from build123d import *

# Parameters (mm, degrees)
F0_W        = 7
F0_H        = 7
F0_W_2      = 1.15
F0_H_2      = 1.15
F1_DEPTH    = 6
F2_SIZE     = 0.1
F3_T1_DEPTH = 14.6069618105
F3_T3_DEPTH = 14.6069618105
F3_T5_DEPTH = 14.6069618105
F3_T7_DEPTH = 14.6069618105
F6_D        = 3
F6_DEPTH    = 6
F6_TIP      = 0.9012909285
F8_DEPTH    = 3.5
F9_SIZE     = 0.3


# Not quite as in the source:
# - a fillet or chamfer that OpenCascade refuses, or shapes differently, is made with other operations: its cross-section is extruded or revolved along the edge and cut away or added


with BuildPart() as f1:
    # F0 (on Front) → F1 (new body)
    with BuildSketch(Plane.XZ):
        Rectangle(F0_W, F0_H)
        with Locations((-2.54, -2.54)):
            Rectangle(F0_W_2, F0_H_2, mode=Mode.SUBTRACT)
        with Locations((0, -2.54)):
            Rectangle(F0_W_2, F0_H_2, mode=Mode.SUBTRACT)
        with Locations((2.54, -2.54)):
            Rectangle(F0_W_2, F0_H_2, mode=Mode.SUBTRACT)
        with Locations((-2.54, 2.54)):
            Rectangle(F0_W_2, F0_H_2, mode=Mode.SUBTRACT)
        with Locations((0, 2.54)):
            Rectangle(F0_W_2, F0_H_2, mode=Mode.SUBTRACT)
        with Locations((2.54, 2.54)):
            Rectangle(F0_W_2, F0_H_2, mode=Mode.SUBTRACT)
        with Locations((-2.54, -2.54)):
            Rectangle(F0_W_2, F0_H_2)
        with Locations((0, -2.54)):
            Rectangle(F0_W_2, F0_H_2)
        with Locations((0, 2.54)):
            Rectangle(F0_W_2, F0_H_2)
        with Locations((-2.54, 2.54)):
            Rectangle(F0_W_2, F0_H_2)
        with Locations((2.54, 2.54)):
            Rectangle(F0_W_2, F0_H_2)
        with Locations((2.54, -2.54)):
            Rectangle(F0_W_2, F0_H_2)
    extrude(amount=F1_DEPTH)

    # F2
    f2_edges = [f1.edges().sort_by_distance(p)[0] for p in [
        (3.5, -6, 0),
        (0, -6, 3.5),
        (-3.5, -6, 0),
        (0, -6, -3.5),
    ]]
    chamfer(f2_edges, length=F2_SIZE)

    # F3: fillet of radius 5 on 4 edges, made by hand

    # F3_s2 → F3_t1 (cut)
    with BuildSketch(Plane(origin=(4.5333333333, 4.5333333333, 4.5333333333), x_dir=(0.7071067812, -0.7071067812, 0), z_dir=(-0.5773502692, -0.5773502692, -0.5773502692))):
        with BuildLine():
            ThreePointArc((4.1468037432, 5.2809096033), (5.9769307621, 3.4507825844), (6.6468037432, 0.9507825844))
            Line((6.6468037432, 0.9507825844), (6.6468037432, 3.8375339304))
            Line((6.6468037432, 3.8375339304), (4.1468037432, 5.2809096033))
        make_face()
    extrude(amount=F3_T1_DEPTH, mode=Mode.SUBTRACT)

    # F3_s4 → F3_t3 (cut)
    with BuildSketch(Plane(origin=(-4.5333333333, 4.5333333333, 4.5333333333), x_dir=(0.7071067812, 0.7071067812, 0), z_dir=(0.5773502692, -0.5773502692, -0.5773502692))):
        with BuildLine():
            ThreePointArc((-4.1468037432, 5.2809096033), (-5.9769307621, 3.4507825844), (-6.6468037432, 0.9507825844))
            Line((-6.6468037432, 0.9507825844), (-6.6468037432, 3.8375339304))
            Line((-6.6468037432, 3.8375339304), (-4.1468037432, 5.2809096033))
        make_face()
    extrude(amount=F3_T3_DEPTH, mode=Mode.SUBTRACT)

    # F3_s6 → F3_t5 (cut)
    with BuildSketch(Plane(origin=(4.5333333333, 4.5333333333, -4.5333333333), x_dir=(0.7071067812, -0.7071067812, 0), z_dir=(-0.5773502692, -0.5773502692, 0.5773502692))):
        with BuildLine():
            ThreePointArc((6.6468037432, -0.9507825844), (5.9769307621, -3.4507825844), (4.1468037432, -5.2809096033))
            Line((4.1468037432, -5.2809096033), (6.6468037432, -3.8375339304))
            Line((6.6468037432, -3.8375339304), (6.6468037432, -0.9507825844))
        make_face()
    extrude(amount=F3_T5_DEPTH, mode=Mode.SUBTRACT)

    # F3_s8 → F3_t7 (cut)
    with BuildSketch(Plane(origin=(-4.5333333333, 4.5333333333, -4.5333333333), x_dir=(0.7071067812, 0.7071067812, 0), z_dir=(0.5773502692, -0.5773502692, 0.5773502692))):
        with BuildLine():
            ThreePointArc((-6.6468037432, -0.9507825844), (-5.9769307621, -3.4507825844), (-4.1468037432, -5.2809096033))
            Line((-4.1468037432, -5.2809096033), (-6.6468037432, -3.8375339304))
            Line((-6.6468037432, -3.8375339304), (-6.6468037432, -0.9507825844))
        make_face()
    extrude(amount=F3_T7_DEPTH, mode=Mode.SUBTRACT)

    # F6
    with Locations(Plane.XZ.offset(6)):
        with Locations((0, 0)):
            Hole(F6_D / 2, depth=F6_DEPTH)
            with Locations((0, 0, -(F6_DEPTH + F6_TIP / 2))):  # 118° drill point
                Cone(0, F6_D / 2, F6_TIP, mode=Mode.SUBTRACT)

    # F0 (on Front) → F8 (join)
    with BuildSketch(Plane.XZ):
        with Locations((2.54, 2.54)):
            Rectangle(F0_W_2, F0_H_2)
        with Locations((0, 2.54)):
            Rectangle(F0_W_2, F0_H_2)
        with Locations((-2.54, 2.54)):
            Rectangle(F0_W_2, F0_H_2)
        with Locations((-2.54, -2.54)):
            Rectangle(F0_W_2, F0_H_2)
        with Locations((0, -2.54)):
            Rectangle(F0_W_2, F0_H_2)
        with Locations((2.54, -2.54)):
            Rectangle(F0_W_2, F0_H_2)
    extrude(amount=-F8_DEPTH)

    # F9
    f9_edges = [f1.edges().sort_by_distance(p)[0] for p in [
        (2.54, 3.5, -3.115),
        (1.965, 3.5, -2.54),
        (3.115, 3.5, -2.54),
        (2.54, 3.5, -1.965),
        (0.575, 3.5, -2.54),
        (0, 3.5, -3.115),
        (-0.575, 3.5, -2.54),
        (0, 3.5, -1.965),
        (-1.965, 3.5, -2.54),
        (-2.54, 3.5, -1.965),
        (-3.115, 3.5, -2.54),
        (-2.54, 3.5, -3.115),
        (3.115, 3.5, 2.54),
        (2.54, 3.5, 1.965),
        (1.965, 3.5, 2.54),
        (2.54, 3.5, 3.115),
        (0.575, 3.5, 2.54),
        (0, 3.5, 3.115),
        (-0.575, 3.5, 2.54),
        (0, 3.5, 1.965),
        (-1.965, 3.5, 2.54),
        (-2.54, 3.5, 1.965),
        (-3.115, 3.5, 2.54),
        (-2.54, 3.5, 3.115),
    ]]
    chamfer(f9_edges, length=F9_SIZE)


solid = f1.part
Input: part model. Units: mm. Frame: model coordinates. A direction names the side the tool comes from. Coordinates: 2 decimals unless noted, no trailing zeros. Loops run counter-clockwise (first coordinate to the right, second up) from the corner with the lowest first, then second, coordinate; pieces in that order, holes last.
(1) Set-up query: faces 5 (the face through (3.115, 1.6, 2.5)), 6 (the face through (1.965, 1.6, -2.5)), 7 (the face through (-3.115, 1.6, 2.5)), 8 (the face through (2.5, 1.6, 1.965)). Return all of +Z, -Z, +X, -X, +Y, -Y with unobstructed straight access to the full face (end or side cutting, diameter ignored); none if empty.
(2) Pull-direction query (X, two-part tool) for faces 1 (the face through (0.575, 1.6, -2.5)), 2 (the face through (3.115, 1.6, -2.5)), 3 (the face through (-2.72, -5.724, 2.737)), 4 (the face through (-2.5, 1.6, -1.965)); classes: released by +X, released by -X, zero draft, split by the parting line, or undercut.
(3) First-contact query: pin 1 Ø0.6 at (y, z) = (1, 2.5) entering from +X (3 decimals); pin 2 Ø0.9 at (x, y) = (0, 1.5) entering from +Z (3 decimals); pin 3 Ø0.6 at (y, z) = (2, 2.5) entering from -X (3 decimals). Flat tips, straight axial feed; report the tip coordinate or a pass-through.
(4) Section B-B on y = -3.5. Return the cut outline in (x, z).
(5) Material intervals for probe 1 along X at (y, z) = (2.25, -2.75) (3 decimals); probe 2 along Z at (x, y) = (0, -3.4); probe 3 along Z at (x, y) = (-2.75, 2.5) (3 decimals), sorted ascending.
(6) Section A-A on y = 0.25. Return the cut outline in (x, z) (3 decimals).
Data:
1. face 5: +Z, -Z, +X, +Y
1. face 6: +Z, -Z, +Y
1. face 7: +Z, -Z, -X, +Y
1. face 8: +X, -X, +Y
2. face 1: undercut
2. face 2: released by +X
2. face 3: released by -X
2. face 4: zero draft
3. pin 1: stops at x = 3.115
3. pin 2: stops at z = 3.115
3. pin 3: stops at x = -3.115
4. outline: (-3.5, -3.5) - (3.5, -3.5) - (3.5, 3.5) - (-3.5, 3.5) - close; hole circle Ø3 at (0, 0)
5. probe 1: x = -3.115 to -1.965, -0.575 to 0.575, 1.965 to 3.115
5. probe 2: z = -3.5 to -1.5, 1.5 to 3.5
5. probe 3: z = -3.115 to -1.965, 1.965 to 3.115
6. outline: (-3.115, -3.115) - (-1.965, -3.115) - (-1.965, -1.965) - (-3.115, -1.965) - close; (-3.115, 1.965) - (-1.965, 1.965) - (-1.965, 3.115) - (-3.115, 3.115) - close; (-0.575, -3.115) - (0.575, -3.115) - (0.575, -1.965) - (-0.575, -1.965) - close; (-0.575, 1.965) - (0.575, 1.965) - (0.575, 3.115) - (-0.575, 3.115) - close; (1.965, -3.115) - (3.115, -3.115) - (3.115, -1.965) - (1.965, -1.965) - close; (1.965, 1.965) - (3.115, 1.965) - (3.115, 3.115) - (1.965, 3.115) - close
